CAD build for the part. Positions are in the model's coordinates, mm. A direction names the side the tool comes from. Coordinates: 2 decimals unless noted, no trailing zeros. Order: outer loops, then holes, each group sorted by start corner. A loop starts at its lowest first (then second) coordinate and runs counter-clockwise, first axis right, second up.
from build123d import *
from build123d.topology import SkipClean

# Parameters (mm, degrees)
BOSS_EXTRUDE1_DEPTH   = 7.5
CUT_EXTRUDE1_DEPTH    = 90.620722002
SKETCH4_R             = 24.5
BOSS_EXTRUDE3_DEPTH   = 50
LPATTERN6_START       = -60.928565373
LPATTERN6_DEPTH       = 11.857130746
LPATTERN6_START_2     = -62.5
LPATTERN6_2_OUTLINE_R = 24.5
LPATTERN6_2_DEPTH     = 15
LPATTERN6_3_OUTLINE_R = 24.5
LPATTERN6_3_DEPTH     = 1.571434627
LPATTERN6_START_3     = -49.996237981
LPATTERN6_4_DEPTH     = 99.992475962
BOSS_EXTRUDE5_DEPTH   = 10
SKETCH8_R             = 30
BOSS_EXTRUDE7_DEPTH   = 20


with BuildPart() as part:
    # Sketch1 → Boss-Extrude1 (new, symmetric)
    with BuildSketch(Plane.XY):
        with BuildLine():
            ThreePointArc((-24.948290112, 50.607115575), (0, 74), (24.948290112, 50.607115575))
            ThreePointArc((24.948290112, 50.607115575), (32.398481343, 25.282941249), (49.996237981, 5.607115575))
            ThreePointArc((49.996237981, 5.607115575), (0, -32.02671366), (-49.996237981, 5.607115575))
            ThreePointArc((-49.996237981, 5.607115575), (-32.398481343, 25.282941249), (-24.948290112, 50.607115575))
        make_face()
    extrude(amount=BOSS_EXTRUDE1_DEPTH, both=True)

    # Sketch2 → Cut-Extrude1 (cut, symmetric)
    with BuildSketch(Plane(origin=(0, 0, 0), x_dir=(0, 0, -1), z_dir=(1, 0, 0))):
        Polygon((-7.5, 29), (-5.928565373, 74), (-7.5, 74), align=None)
        Polygon((7.5, 74), (7.5, 29), (5.928565373, 74), align=None)
    extrude(amount=CUT_EXTRUDE1_DEPTH, both=True, mode=Mode.SUBTRACT)

    # Sketch4 → Boss-Extrude3 (add)
    with BuildSketch(Plane.XY):
        with Locations((0, 49)):
            Circle(SKETCH4_R)
    extrude(amount=-BOSS_EXTRUDE3_DEPTH)

    # LPattern6: read off the stored shape, not the designer's step
    # LPattern6 outline → LPattern6 (add)
    with BuildSketch(Plane.XY.offset(LPATTERN6_START)):
        with BuildLine():
            ThreePointArc((-49.996237981, 5.607115575), (0, -32.02671366), (49.996237981, 5.607115575))
            ThreePointArc((49.996237981, 5.607115575), (32.398481343, 25.282941249), (24.948290112, 50.607115575))
            ThreePointArc((24.948290112, 50.607115575), (0, 74), (-24.948290112, 50.607115575))
            ThreePointArc((-24.948290112, 50.607115575), (-32.398481343, 25.282941249), (-49.996237981, 5.607115575))
        make_face()
    extrude(amount=LPATTERN6_DEPTH)

    # LPattern6 2 outline → LPattern6 2 (add)
    with BuildSketch(Plane.XY.offset(LPATTERN6_START_2)):
        with BuildLine():
            ThreePointArc((-49.996237981, 5.607115575), (0, -32.02671366), (49.996237981, 5.607115575))
            ThreePointArc((49.996237981, 5.607115575), (32.398481343, 25.282941249), (24.948290112, 50.607115575))
            ThreePointArc((24.948290112, 50.607115575), (0, 74), (-24.948290112, 50.607115575))
            ThreePointArc((-24.948290112, 50.607115575), (-32.398481343, 25.282941249), (-49.996237981, 5.607115575))
        make_face()
        with Locations((0, 49)):
            Circle(LPATTERN6_2_OUTLINE_R, mode=Mode.SUBTRACT)
    extrude(amount=LPATTERN6_2_DEPTH)

    # LPattern6 3 outline → LPattern6 3 (add)
    with BuildSketch(Plane.XY.offset(LPATTERN6_START_2)):
        with Locations((0, 49)):
            Circle(LPATTERN6_3_OUTLINE_R)
    extrude(amount=LPATTERN6_3_DEPTH)

    # LPattern6 4 outline → LPattern6 4 (cut)
    with BuildSketch(Plane.YZ.offset(LPATTERN6_START_3)):
        Polygon((75, -60.893644604), (74, -60.928565373), (29, -62.5), (75, -62.5), align=None)
        Polygon((74, -49.071434627), (75, -49.106355396), (75, -47.5), (29, -47.5), align=None)
    extrude(amount=LPATTERN6_4_DEPTH, mode=Mode.SUBTRACT)

    # Sketch5 → Boss-Extrude5 (add)
    with SkipClean():  # the faces are left unmerged after this step: merging them gives an invalid solid
        with BuildSketch(Plane(origin=(0, 0, -47.5), x_dir=(-1, 0, 0), z_dir=(0, 0, -1))):
            with BuildLine():
                Line((-14.150971698, 29), (14.150971698, 29))
                ThreePointArc((14.150971698, 29), (0, 73.5), (-14.150971698, 29))
            make_face()
        extrude(amount=BOSS_EXTRUDE5_DEPTH)

    # Sketch8 → Boss-Extrude7 (add)
    with SkipClean():  # the faces are left unmerged after this step: merging them gives an invalid solid
        with BuildSketch(Plane(origin=(0, 0, -62.5), x_dir=(-1, 0, 0), z_dir=(0, 0, -1))):
            with Locations(Location((0, 0, 0), (0, 0, 104.835111582))):
                Circle(SKETCH8_R)
        extrude(amount=BOSS_EXTRUDE7_DEPTH)


solid = part.part
1) Two-plate mould, pull along Z, no slides. Class faces 1 (the flat face through (-1, -1, -47.5)), 2 (the flat face through (1, -1, -7.5)), 3 (the cylindrical face through (0.94, -32.02, 0.11)), 4 (the flat face through (0, -1, -82.5)): released by +Z, released by -Z, zero draft, split by the parting line, or undercut.
2) Slice it at B-B (y = -11.5). List the corners of the cut face in (x, z), plus the area to 3 significant figures.
3) Slice it at D-D (z = -33.5). List the corners of the cut face in (x, y), plus the area to 3 significant figures.
4) Drill centre lines: probe 1 along Z at (x, y) = (-17.5, -5); probe 2 along Z at (x, y) = (29.5, 27); probe 3 along X at (y, z) = (38.5, -13.5). Where is each one in solid material? Low to high.
5) Which spindle directions (+Z, -Z, +X, -X, +Y, -Y) get a long thin tool onto all of the face, cutting with end or side? Do faces 5 (the cylindrical face through (32.22, 25.61, 0.11)), 6 (the cylindrical face through (27.753, -11.391, -72.36)). Say none if no direction does.
6) Slice it at C-C (x = 35). List the corners of the cut face in (y, z), plus the area to 3 significant figures.
7) Pin check, flat tips, straight feed: P1, Ø8, axis at y = -6, z = -7, coming from the -X side; P2, Ø1.5, axis at x = 6, z = -36, coming from the -Y side; P3, Ø1.5, axis at x = 22, y = 38.5, coming from the +Z side; P4, Ø1.5, axis at x = 33, z = -46, coming from the +Y side. Stop position of each tip, or through.
8) Slice it at A-A (x = 0). List the corners of the cut face in (y, z).
Worked out:
1. face 1: undercut
1. face 2: undercut
1. face 3: zero draft
1. face 4: released by -Z
2. outline: (-41.41, -62.5) - (-27.71, -62.5) - (-27.71, -82.5) - (27.71, -82.5) - (27.71, -62.5) - (41.41, -62.5) - (41.41, -47.5) - (-41.41, -47.5) - close; (-41.41, -7.5) - (41.41, -7.5) - (41.41, 7.5) - (-41.41, 7.5) - close
2. area: 3,590 mm2
3. outline: circle Ø49 at (0, 49)
3. area: 1,890 mm2
4. probe 1: z = -82.5 to -47.5, -7.5 to 7.5
4. probe 2: z = -62.5 to -47.5, -7.5 to 7.5
4. probe 3: x = -22.14 to 22.14
5. face 5: +Z, -Z, +X, +Y
5. face 6: -Z
6. outline: (-18.49, -62.5) - (21.03, -62.5) - (21.03, -47.5) - (-18.49, -47.5) - close; (-18.49, -7.5) - (21.03, -7.5) - (21.03, 7.5) - (-18.49, 7.5) - close
6. area: 1,190 mm2
7. P1: stops at x = -47.15
7. P2: stops at y = 25.07
7. P3: stops at z = 7.19
7. P4: passes through
8. outline: (-32.03, -62.5) - (-30, -62.5) - (-30, -82.5) - (30, -82.5) - (30, -62.5) - (29, -62.5) - (74, -60.93) - (74, -49.07) - (73.5, -49.05) - (73.5, -5.95) - (74, -5.93) - (74, 5.93) - (29, 7.5) - (-32.03, 7.5) - (-32.03, -7.5) - (24.5, -7.5) - (24.5, -47.5) - (-32.03, -47.5) - close
